from build123d import *

# Parameters (mm, degrees)
F1_DEPTH = 50
F2_R     = 5


with BuildPart() as f1:
    # F0 (on Front) → F1 (new body)
    with BuildSketch(Plane.XZ):
        Polygon((0, 40), (0, 0), (60, 0), (60, 10), (27.063251, 10), (10, 20.432902), (10, 40), align=None)
    extrude(amount=-F1_DEPTH)

    # F2
    f2_edges = [f1.edges().sort_by_distance(p)[0] for p in [
        (5, 0, 40),
        (5, 50, 40),
        (60, 0, 5),
        (60, 50, 5),
    ]]
    fillet(f2_edges, radius=F2_R)


solid = f1.part
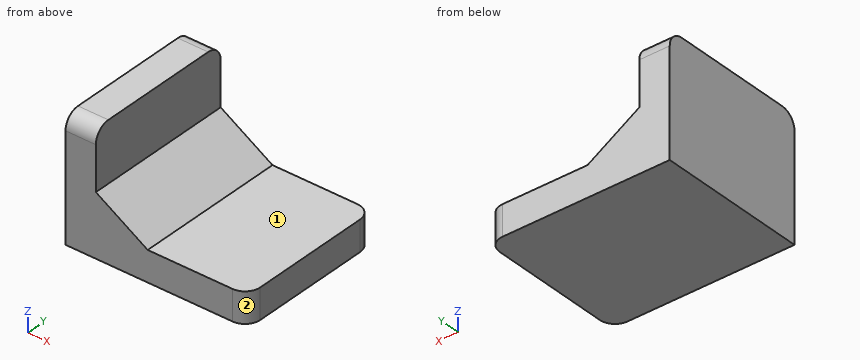
Here's how the part is built. I have some questions about the finished solid (model axes, mm). Face numbers are marked on the shaded views. A direction names the side the tool comes from. Coordinates: 2 decimals unless noted, no trailing zeros. Write each loop counter-clockwise with the first axis right and the second up, starting at its lowest first coordinate (ties: lowest second). Pieces come first, ordered by that corner, then holes.
1) Which directions (+Z, -Z, +X, -X, +Y, -Y) give clear straight access to the entire face, cutting with the end or side of a thin tool? Please do the marked faces 1 and 2.
Filled in:
face 1: +Z, +X, +Y, -Y
face 2: +Z, -Z, +X, -Y
2) If we section it at C-C (z = 28.5): List the corners of the cut face in (x, y) for me.
Filled in:
outline: (0, 0) - (10, 0) - (10, 50) - (0, 50) - close
3) I'm going to push flat-ended pins straight in: pin 1 (1.5 mm diameter, centred on x = 40, y = 23.5, fed in from -Z); pin 2 (4 mm diameter, centred on y = 21.5, z = 22.5, fed in from +X); pin 3 (16.5 mm diameter, centred on x = 43, y = 18.5, fed in from +Z); pin 4 (1 mm diameter, centred on x = 53, z = 11.5, fed in from -Y). Where does each tip first touch, or does it pass through?
Filled in:
pin 1: stops at z = 0
pin 2: stops at x = 10
pin 3: stops at z = 10
pin 4: passes through
4) If we section it at D-D (y = 4): List the corners of the cut face in (x, z) for me, plus the area to 3 significant figures.
Filled in:
outline: (0, 0) - (59.9, 0) - (59.9, 10) - (27.06, 10) - (10, 20.43) - (10, 39.9) - (0, 39.9) - close
area: 987 mm2
5) If I drill on line 1 (X direction, y = 20.5, z = 33); line 2 (X direction, y = 4.5, z = 15.5), over which ranges is the centre line in solid material (lowest first)?
Filled in:
line 1: x = 0 to 10
line 2: x = 0 to 18.07
6) If we section it at A-A (y = 13.5): List the corners of the cut face in (x, z) for me, plus the area to 3 significant figures.
Filled in:
outline: (0, 0) - (60, 0) - (60, 10) - (27.06, 10) - (10, 20.43) - (10, 40) - (0, 40) - close
area: 989 mm2
7) If we section it at B-B (x = 29): List the corners of the cut face in (y, z) for me.
Filled in:
outline: (0, 0) - (50, 0) - (50, 10) - (0, 10) - close
